Could you check a few things on this model? Use its own coordinates, in mm. A direction names the side the tool comes from. Give positions to 0.01 mm unless a question says otherwise; leave off trailing zeros. Loops run counter-clockwise (first coordinate to the right, second up) from the corner with the lowest first, then second, coordinate; pieces in that order, holes last. Notation, with made-up numbers: M -1,51.25 L 12,51.25 A23 ccw 12,83.25 Z; hole C -30.75,28 d5. An arc over 180 degrees is marked long. Write each question's results on one line, items separated by ' | '. Start each with the question number.
from build123d import *

# Parameters (mm, degrees)
ESBO_O1_R                = 3.5
RESSALTO_EXTRUS_O1_DEPTH = 10
ESBO_O3_W                = 13
ESBO_O3_H                = 18
CORTE_EXTRUS_O2_DEPTH    = 10
ESBO_O4_R                = 5
RESSALTO_EXTRUS_O2_DEPTH = 100


with BuildPart() as part:
    # Esboço1 → Ressalto-extrusão1 (new, symmetric)
    with BuildSketch(Plane(origin=(0, 0, 0), x_dir=(0, 0, -1), z_dir=(1, 0, 0))):
        with BuildLine():
            Line((-6, 0), (-6, -22))
            Line((-6, -22), (6, -22))
            Line((6, -22), (6, 0))
            ThreePointArc((6, 0), (0, 6), (-6, 0))
        make_face()
        Circle(ESBO_O1_R, mode=Mode.SUBTRACT)
    extrude(amount=RESSALTO_EXTRUS_O1_DEPTH, both=True)

    # Esboço3 → Corte-extrusão2 (cut, symmetric)
    with BuildSketch(Plane.XY):
        with Locations((0, -3)):
            Rectangle(ESBO_O3_W, ESBO_O3_H)
    extrude(amount=CORTE_EXTRUS_O2_DEPTH, both=True, mode=Mode.SUBTRACT)

    # Esboço4 → Ressalto-extrusão2 (add)
    with BuildSketch(Plane.XZ.offset(22)):
        with Locations(Location((0, 0, 0), (0, 0, 90))):
            Circle(ESBO_O4_R)
    extrude(amount=RESSALTO_EXTRUS_O2_DEPTH)


solid = part.part
1) Which directions (+Z, -Z, +X, -X, +Y, -Y) give clear straight access to the entire face, cutting with the end or side of a thin tool? Please do faces 1 (the face through (6.5, -5, 0)), 2 (the face through (10, -11, 0)), 3 (the face through (4.88, -71.3, -1.08)).
2) If we section it at D-D on y = -104: Write out the boundary of the cut face in (x, z).
3) If we section it at B-B on x = 3: Write out the boundary of the cut face in (y, z), plus the area to 3 significant figures.
4) Please list where these lines run through material, in increasing order: line 1 (Y direction, x = -7.75, z = 0); line 2 (Z direction, x = 7.85, y = 0); line 3 (Y direction, x = 4.5, z = -2.25). Write a range as from..to.
5) If we section it at A-A on z = 0: Write out the boundary of the cut face in (x, y), plus the area to 3 significant figures.
6) Thinking about a two-plate mould opening in Y: for faces 4 (the face through (0, -13, 6)), 5 (the face through (-8, 6, 0)), 6 (the face through (8.226, -1.341, -3.233)), 7 (the face through (-8.274, -1.341, -3.233)), which applies, pulls with the +Y half, pulls with the -Y half, needs draft (parallel to the pull), parting line crosses it, or undercut?
7) I'm going to push flat-ended pins straight in: P1, Ø3, axis at y = -44.5, z = -1.5, coming from the -X side; P2, Ø4, axis at y = -52, z = 1, coming from the +X side; P3, Ø5, axis at x = 4.5, y = -45, coming from the +Z side. Where does each tip first touch, or does it pass through?
8) If we section it at C-C on x = 8.75: Write out the boundary of the cut face in (y, z).
Calculated:
1) face 1: +Z, -Z, +Y | face 2: +Z, -Z, +X, +Y, -Y | face 3: -Y
2) outline: C 0,0 d10
3) outline: M -122,-4 L -22,-4 L -22,-6 L -12,-6 L -12,6 L -22,6 L -22,4 L -122,4 Z | area: 920 mm2
4) line 1: y = -22..-3.5, 3.5..6 | line 2: z = -6..-3.5, 3.5..6 | line 3: y = -22..-12
5) outline: M -10,-22 L -5,-22 L -5,-122 L 5,-122 L 5,-22 L 10,-22 L 10,-3.5 L 6.5,-3.5 L 6.5,-12 L -6.5,-12 L -6.5,-3.5 L -10,-3.5 Z; M -10,3.5 L -6.5,3.5 L -6.5,6 L -10,6 Z; M 6.5,3.5 L 10,3.5 L 10,6 L 6.5,6 Z | area: 1,280 mm2
6) face 4: needs draft | face 5: pulls with the +Y half | face 6: undercut | face 7: undercut
7) P1: stops at x = -5 | P2: stops at x = 5 | P3: stops at z = 4.58
8) outline: M -22,-6 L 0,-6 A6 ccw 0,6 L -22,6 Z; hole C 0,0 d7
